Here's how the part is built. I have some questions about the finished solid (model axes, mm). A direction names the side the tool comes from. Give positions to 0.01 mm unless a question says otherwise; leave off trailing zeros. Loops run counter-clockwise (first coordinate to the right, second up) from the corner with the lowest first, then second, coordinate; pieces in that order, holes last.
Q1. If we section it at D-D (z = -131): Please give me the cut outline in (x, y).
Q2. If we section it at A-A (y = 5): Give the number of separate pieces and of enclosed holes in the cut face, plus the area to 3 significant figures.
Q3. For faces 1 (the face through (21, 0, -85)), 2 (the face through (7.553, 4.93, -119.924)), 3 (the face through (16.756, 5.068, -2.535)), 4 (the face through (2.535, 4.406, -27.592)), which set-ups out of +Z, -Z, +X, -X, +Y, -Y let a thin tool reach every point of the face, with its end or its side?
Q4. We'd pull the mould along Z, two halves only. Please class faces 5 (the face through (25.833, 4.93, -100.386)), 6 (the face through (0, 3, -98)), 7 (the face through (23, 5, -5)): +Z half, -Z half, draft (parallel to the pull), parting line (faces both ways), or undercut.
Q5. I need wall thicknesses on line 1 (Y direction, x = 1, z = -26); line 2 (X direction, y = 6, z = -31); line 3 (X direction, y = 9.25, z = -62.5). Which ranges of each line are inside material? Lowest first, please.
Q6. If we section it at C-C (x = 48.5): Please give me the cut outline in (y, z).
Q7. If we section it at B-B (z = -34): Please give me the cut outline in (x, y).
Q8. Will these pins go through, and if not, where does the flat tip stop? P1, Ø4, axis at y = 5, z = -53.4, coming from the -X side; P2, Ø2.5, axis at y = 5, z = -71.56, coming from the +X side; P3, Ø1.9, axis at y = 5, z = -98.8, coming from the +X side; P4, Ø2, axis at y = 6, z = -76.5, coming from the +X side.
from build123d import *

# Parameters (mm, degrees)
BOSS_EXTRUDE1_DEPTH = 10
SKETCH2_R           = 1.55
CUT_EXTRUDE1_DEPTH  = 7
SKETCH3_R           = 1.55
CUT_EXTRUDE2_DEPTH  = 7


with BuildPart() as part:
    # Sketch1 → Boss-Extrude1 (new body)
    with BuildSketch(Plane(origin=(0, 0, 0), x_dir=(1, 0, 0), z_dir=(0, 1, 0))):
        Polygon((0, 0), (0, 198), (52.4, 0), align=None)
        with BuildLine():
            Line((5, 8), (5, 116.957761971))
            ThreePointArc((5, 116.957761971), (7.613008346, 119.932696838), (10.900158307, 117.725278614))
            Line((10.900158307, 117.725278614), (39.735444808, 8.767516643))
            ThreePointArc((39.735444808, 8.767516643), (39.212527542, 6.170047805), (36.835286501, 5))
            Line((36.835286501, 5), (8, 5))
            ThreePointArc((8, 5), (5.878679656, 5.878679656), (5, 8))
        make_face(mode=Mode.SUBTRACT)
    extrude(amount=BOSS_EXTRUDE1_DEPTH)

    # Sketch2 → Cut-Extrude1 (cut)
    with BuildSketch(Plane(origin=(0, 0, -5), x_dir=(-1, 0, 0), z_dir=(0, 0, -1))):
        with Locations((-15.207643251, 5)):
            Circle(SKETCH2_R)
        with Locations((-29.627643251, 5)):
            Circle(SKETCH2_R)
    extrude(amount=-CUT_EXTRUDE1_DEPTH, mode=Mode.SUBTRACT)

    # Sketch3 → Cut-Extrude2 (cut)
    with BuildSketch(Plane(origin=(5, 0, 0), x_dir=(0, 0, -1), z_dir=(1, 0, 0))):
        with Locations((98.797761971, 5)):
            Circle(SKETCH3_R)
        with Locations((71.557761971, 5)):
            Circle(SKETCH3_R)
        with Locations((53.4, 5)):
            Circle(SKETCH3_R)
        with Locations((26.16, 5)):
            Circle(SKETCH3_R)
    extrude(amount=-CUT_EXTRUDE2_DEPTH, mode=Mode.SUBTRACT)


solid = part.part
Check sheet entries:
1. outline: (0, 0) - (17.73, 0) - (17.73, 10) - (0, 10) - close
2. separate pieces: 6
2. enclosed holes: 0
2. area: 2,740 mm2
3. face 1: +Z, -Z, +X, -X, -Y
3. face 2: +Y, -Y
3. face 3: +Z
3. face 4: -X
4. face 5: -Z half
4. face 6: draft
4. face 7: undercut
5. line 1: y = 0 to 3.46, 6.54 to 10
5. line 2: x = 0 to 5, 33.85 to 44.2
5. line 3: x = 0 to 5, 25.52 to 35.86
6. outline: (0, -14.74) - (10, -14.74) - (10, 0) - (0, 0) - close
7. outline: (0, 0) - (5, 0) - (5, 10) - (0, 10) - close; (33.06, 0) - (43.4, 0) - (43.4, 10) - (33.06, 10) - close
8. P1: stops at x = 0
8. P2: stops at x = 33.79
8. P3: stops at x = 26.5
8. P4: stops at x = 32.42
